Design review of the part built by this model. Coordinates are the model's own, in mm. Coordinates: 2 decimals unless noted, no trailing zeros. Write each loop counter-clockwise with the first axis right and the second up, starting at its lowest first coordinate (ties: lowest second). Pieces come first, ordered by that corner, then holes. Notation, with made-up numbers: (71.5, 49) -> (81.5, 49) arc R37 cw to (81.5, 87) -> close; hole circle Ø11 at (54, 55). An arc over 180 degrees is marked (long way). Answer in a Markdown table with one row per item. Add a question column.
Item 1: To check wall thickness, follow line 1 (Z direction, x = 1.25, y = -2.75) (3 decimals); line 2 (Z direction, x = -3, y = 0.5) (3 decimals); line 3 (X direction, y = 1.25, z = -71.5). State the ranges of each line that lie inside material, in increasing order.
Item 2: Clearance check with flat-ended pins moving along their axes: P1, Ø1, axis at x = 1, z = -73, coming from the +Y side; P2, Ø3, axis at x = 2.5, z = -66.5, coming from the -Y side. State where each tip first meets the part, or that it passes through.
Item 3: Take a section at A-A, the plane z = -71. Write out the cut boundary in (x, y) (3 decimals), and give its area (3 significant figures).
from build123d import *

# Parameters (mm, degrees)
SKETCH3_R           = 3.175
BOSS_EXTRUDE1_DEPTH = 76.2
CHAMFER1_SIZE       = 0.635
CUT_TO_LENGTH_START = -19.05
SKETCH4_R           = 3.175
CUT_TO_LENGTH_DEPTH = 134.416131485
CHAMER_CUT_END_SIZE = 0.635
SKETCH5_W           = 0.254
SKETCH5_H           = 0.7366


with BuildPart() as part:
    # Sketch3 → Boss-Extrude1 (new, symmetric)
    with BuildSketch(Plane.XY):
        with Locations(Location((0, 0, 0), (0, 0, 180))):
            Circle(SKETCH3_R)
    extrude(amount=BOSS_EXTRUDE1_DEPTH, both=True)

    # Chamfer1
    chamfer1_edges = [part.edges().sort_by_distance(p)[0] for p in [
        (3.175, 0, -76.2),
        (3.175, 0, 76.2),
    ]]
    chamfer(chamfer1_edges, length=CHAMFER1_SIZE)

    # Sketch4 → CUT-TO-LENGTH (cut, through all)
    with BuildSketch(Plane(origin=(0, 0, -76.2), x_dir=(-1, 0, 0), z_dir=(0, 0, -1)).offset(CUT_TO_LENGTH_START)):
        Circle(SKETCH4_R)
    extrude(amount=-CUT_TO_LENGTH_DEPTH, mode=Mode.SUBTRACT)

    # CHAMER-CUT-END
    chamer_cut_end_edges = [part.edges().sort_by_distance(p)[0] for p in [
        (3.175, 0, -57.15),
    ]]
    chamfer(chamer_cut_end_edges, length=CHAMER_CUT_END_SIZE)

    # Sketch5 → SNAP-RING-CUT (revolve, cut)
    with BuildSketch(Plane(origin=(0, 0, 0), x_dir=(1, 0, 0), z_dir=(0, 1, 0))):
        with Locations((3.048, 59.9567)):
            Rectangle(SKETCH5_W, SKETCH5_H)
        with Locations((3.048, 73.3933)):
            Rectangle(SKETCH5_W, SKETCH5_H)
    revolve(axis=Axis((0, 0, -57.785), (0, 0, -1)), mode=Mode.SUBTRACT)


solid = part.part
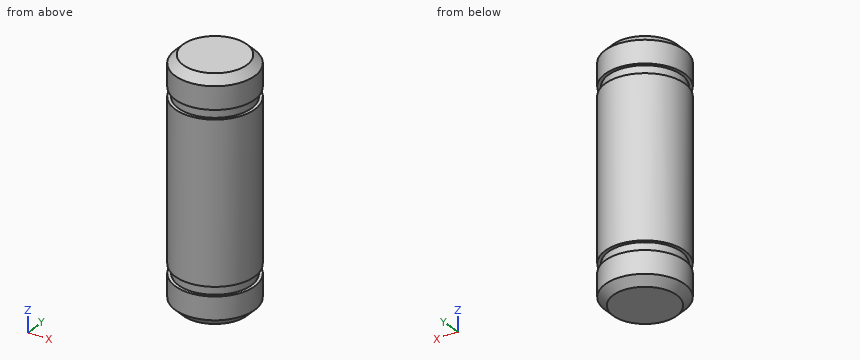
Answers:
| question | item | result |
|---|---|---|
| 1 | line 1 | z = -75.719 to -73.762, -73.025 to -60.325, -59.588 to -57.631 |
| 1 | line 2 | z = -75.699 to -73.762, -73.025 to -60.325, -59.588 to -57.651 |
| 1 | line 3 | x = -2.92 to 2.92 |
| 2 | P1 | stops at y = 3.14 |
| 2 | P2 | stops at y = -3.01 |
| 3 | outline | circle Ø6.35 at (0, 0) |
| 3 | area | 31.7 mm^2 |
